Source: three-view drawing plus pictorial views. Frame: mm from the lowest corner of the part. A direction names the side the tool comes from. Round coordinates to 2 decimals unless told otherwise and drop trailing zeros. Loops run counter-clockwise (first coordinate to the right, second up) from the corner with the lowest first, then second, coordinate; pieces in that order, holes last. Notation, with made-up numbers: (43, 8) -> (74, 8) arc R29 ccw to (74, 40) -> close; hole circle Ø2 at (87, 37). An arc over 180 degrees is marked (long way). Answer as a JSON object with one key per item and string values. Group by question number.
Item 1: Section query C-C on z = 4. Return loops of the section in (x, y), and give its area (3 significant figures).
Item 2: Section query B-B on x = 20. Return loops of the section in (y, z).
Item 3: Section query A-A on x = 4. Return loops of the section in (y, z), and give its area (3 significant figures).
Item 4: Section query D-D on y = 11.5. Return loops of the section in (x, z).
Item 5: Pin query (flat end, axial travel): pin 1 (2 mm diameter, centred on x = 19.5, y = 19, fed in from -Z); pin 2 (3.5 mm diameter, centred on x = 36, z = 20, fed in from +Y); pin 3 (5 mm diameter, centred on x = 26, y = 6, fed in from +Z); pin 4 (5 mm diameter, centred on x = 20, y = 27.69, fed in from +Z). Return the tip coordinate at first contact, or that it passes through.
Item 6: Material intervals for line 1 (X direction, y = 12, z = 25.5) (1 decimal); line 2 (X direction, y = 22, z = 20); line 3 (X direction, y = 7, z = 4), sorted ascending. Write a range as [from, to].
Item 7: Set-up query: the marked faces 1 and 2. Return all of +Z, -Z, +X, -X, +Y, -Y with unobstructed straight access to the full face (end or side cutting, diameter ignored); none if empty.
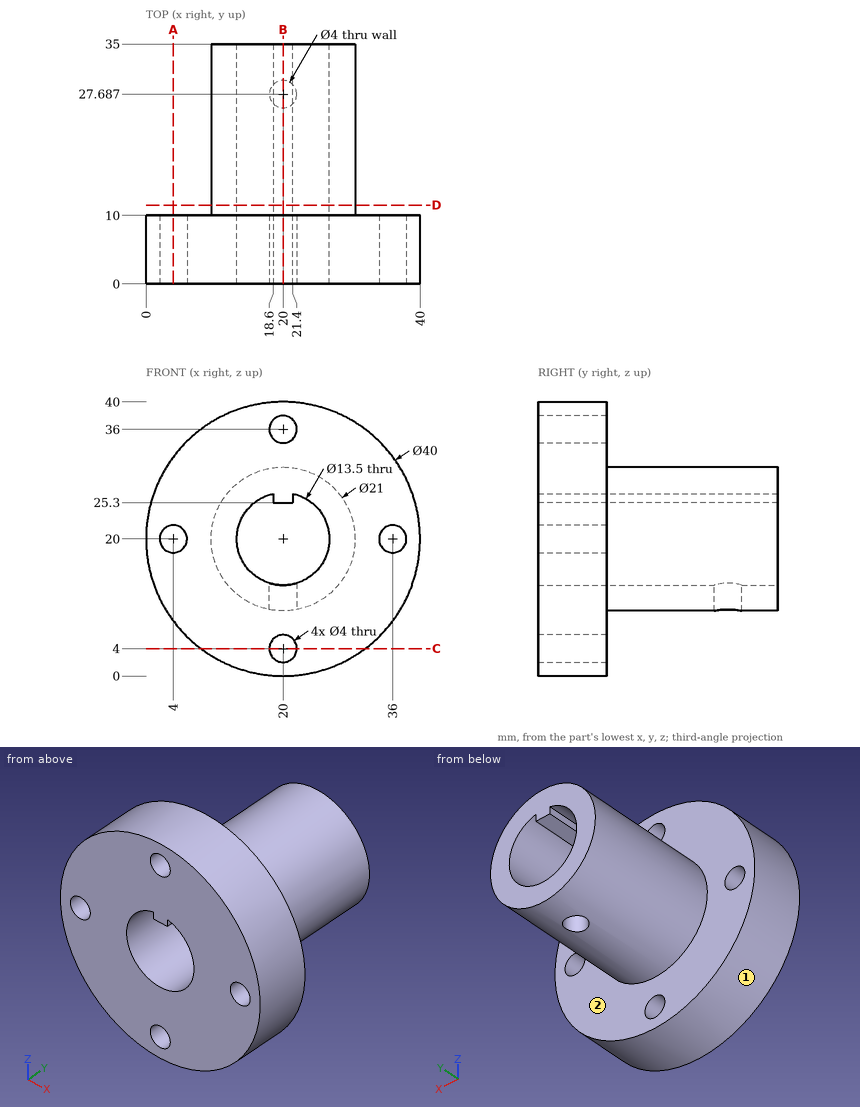
Solved:
{
 "1": {"outline": "(8, 0) -> (18, 0) -> (18, 10) -> (8, 10) -> close; (22, 0) -> (32, 0) -> (32, 10) -> (22, 10) -> close", "area": "200 mm²"},
 "2": {"outline": "(0, 0) -> (10, 0) -> (10, 2) -> (0, 2) -> close; (0, 6) -> (10, 6) -> (10, 9.5) -> (25.69, 9.5) -> (25.69, 13.25) -> (0, 13.25) -> close; (0, 25.3) -> (35, 25.3) -> (35, 30.5) -> (10, 30.5) -> (10, 34) -> (0, 34) -> close; (0, 38) -> (10, 38) -> (10, 40) -> (0, 40) -> close; (29.69, 9.5) -> (35, 9.5) -> (35, 13.25) -> (29.69, 13.25) -> close"},
 "3": {"outline": "(0, 8) -> (10, 8) -> (10, 18) -> (0, 18) -> close; (0, 22) -> (10, 22) -> (10, 32) -> (0, 32) -> close", "area": "200 mm²"},
 "4": {"outline": "circle Ø21 at (20, 20); hole (18.6, 25.3) -> (18.6, 26.6) arc R6.75 ccw (long way) to (21.4, 26.6) -> (21.4, 25.3) -> close"},
 "5": {"pin 1": "z = 9.5", "pin 2": "through", "pin 3": "z = 39.69", "pin 4": "z = 30.5"},
 "6": {"line 1": "[11.1, 16.1], [18.6, 21.4], [23.9, 28.9]", "line 2": "[9.5, 13.25], [26.75, 30.5]", "line 3": "[8, 18], [22, 32]"},
 "7": {"face 1": "+Y, -Y", "face 2": "+Y"}
}
